```python
from build123d import *

# Parameters (mm, degrees)
F0_W     = 70
F0_H     = 21.5599828357
F0_R     = 2.5
F1_DEPTH = 4
F3_DEPTH = 2
F4_R     = 2


with BuildPart() as f1:
    # F0 (on Top) → F1 (new body)
    with BuildSketch(Plane.XY):
        with Locations((18.8872945234, 0.0549508259)):
            Rectangle(F0_W, F0_H)
        with Locations((-9.1127054766, 0)):
            Circle(F0_R, mode=Mode.SUBTRACT)
    extrude(amount=F1_DEPTH)

    # F2 (on face) → F3 (join)
    with BuildSketch(Plane.XY.offset(4)):
        Polygon((2.2051139605, -3.5713818915), (2.8492078737, -5.2161419195), (3.4717942573, -5.2161419195), (1.4376347458, -0.0226395049), (0.9316418122, -0.0226395049), (-1.1127054766, -5.2161419195), (-0.5037027959, -5.2161419195), (0.1324672907, -3.5713818915), align=None)
        with BuildLine():
            Line((1.4161272162, -1.4274207814), (2.0183380454, -3.0302977254))
            Line((2.0183380454, -3.0302977254), (0.3452786363, -3.0302977254))
            Line((0.3452786363, -3.0302977254), (0.9531493418, -1.4274207814))
            add(Edge.make_bspline(
                [(1.1761484646, -0.6814490963), (1.0980421729, -1.0210416691), (0.9531493418, -1.4274207814)],
                knots=[0, 0, 0, 1, 1, 1], degree=2))
            add(Edge.make_bspline(
                [(1.4161272162, -1.4274207814), (1.2995337661, -1.122919441), (1.1761484646, -0.6814490963)],
                knots=[0, 0, 0, 1, 1, 1], degree=2))
        make_face(mode=Mode.SUBTRACT)
        with BuildLine():
            add(Edge.make_bspline(
                [(7.1009068862, -3.8396600241), (7.1009068862, -4.5222410956), (6.6056677174, -4.9048487277)],
                knots=[0, 0, 0, 1, 1, 1], degree=2))
            add(Edge.make_bspline(
                [(6.7952735706, -2.9770948889), (7.1009068862, -3.3098956104), (7.1009068862, -3.8396600241)],
                knots=[0, 0, 0, 1, 1, 1], degree=2))
            add(Edge.make_bspline(
                [(5.6757500553, -2.3545085053), (6.489640255, -2.6442941675), (6.7952735706, -2.9770948889)],
                knots=[0, 0, 0, 1, 1, 1], degree=2))
            add(Edge.make_bspline(
                [(4.9558138008, -2.0381214249), (5.1912646514, -2.1813162932), (5.6757500553, -2.3545085053)],
                knots=[0, 0, 0, 1, 1, 1], degree=2))
            add(Edge.make_bspline(
                [(4.6213151165, -1.7228663198), (4.7203629503, -1.8949265567), (4.9558138008, -2.0381214249)],
                knots=[0, 0, 0, 1, 1, 1], degree=2))
            add(Edge.make_bspline(
                [(4.5222672828, -1.2825279503), (4.5222672828, -1.5508060828), (4.6213151165, -1.7228663198)],
                knots=[0, 0, 0, 1, 1, 1], degree=2))
            add(Edge.make_bspline(
                [(4.791111403, -0.7131444031), (4.5222672828, -0.918031922), (4.5222672828, -1.2825279503)],
                knots=[0, 0, 0, 1, 1, 1], degree=2))
            add(Edge.make_bspline(
                [(5.5376490757, -0.5082568841), (5.0599555232, -0.5082568841), (4.791111403, -0.7131444031)],
                knots=[0, 0, 0, 1, 1, 1], degree=2))
            add(Edge.make_bspline(
                [(6.7828218429, -0.7765350167), (6.1421238554, -0.5082568841), (5.5376490757, -0.5082568841)],
                knots=[0, 0, 0, 1, 1, 1], degree=2))
            Line((6.7828218429, -0.7765350167), (6.9707297333, -0.2535624544))
            add(Edge.make_bspline(
                [(5.5523647539, 0.0294313563), (6.3232398943, 0.0294313563), (6.9707297333, -0.2535624544)],
                knots=[0, 0, 0, 1, 1, 1], degree=2))
            add(Edge.make_bspline(
                [(4.3632247612, -0.3243109071), (4.812052945, 0.0294313563), (5.5523647539, 0.0294313563)],
                knots=[0, 0, 0, 1, 1, 1], degree=2))
            add(Edge.make_bspline(
                [(3.9143965773, -1.2757360988), (3.9143965773, -0.6780531705), (4.3632247612, -0.3243109071)],
                knots=[0, 0, 0, 1, 1, 1], degree=2))
            add(Edge.make_bspline(
                [(4.2239918063, -2.1988619094), (3.9143965773, -1.845119646), (3.9143965773, -1.2757360988)],
                knots=[0, 0, 0, 1, 1, 1], degree=2))
            add(Edge.make_bspline(
                [(5.254655265, -2.8106945282), (4.5335870352, -2.5526041728), (4.2239918063, -2.1988619094)],
                knots=[0, 0, 0, 1, 1, 1], degree=2))
            add(Edge.make_bspline(
                [(6.0238324426, -3.1395333363), (5.7708359758, -2.9940745176), (5.254655265, -2.8106945282)],
                knots=[0, 0, 0, 1, 1, 1], degree=2))
            add(Edge.make_bspline(
                [(6.3849325451, -3.4564864043), (6.2768289094, -3.284992155), (6.0238324426, -3.1395333363)],
                knots=[0, 0, 0, 1, 1, 1], degree=2))
            add(Edge.make_bspline(
                [(6.4930361808, -3.8962587862), (6.4930361808, -3.6279806536), (6.3849325451, -3.4564864043)],
                knots=[0, 0, 0, 1, 1, 1], degree=2))
            add(Edge.make_bspline(
                [(6.1885348404, -4.5318628851), (6.4930361808, -4.3037698737), (6.4930361808, -3.8962587862)],
                knots=[0, 0, 0, 1, 1, 1], degree=2))
            add(Edge.make_bspline(
                [(5.282954646, -4.7599558966), (5.8840335, -4.7599558966), (6.1885348404, -4.5318628851)],
                knots=[0, 0, 0, 1, 1, 1], degree=2))
            add(Edge.make_bspline(
                [(4.5403788867, -4.6818496048), (4.9150626921, -4.7599558966), (5.282954646, -4.7599558966)],
                knots=[0, 0, 0, 1, 1, 1], degree=2))
            add(Edge.make_bspline(
                [(3.8464780628, -4.4701702344), (4.1656950813, -4.603743313), (4.5403788867, -4.6818496048)],
                knots=[0, 0, 0, 1, 1, 1], degree=2))
            Line((3.8464780628, -4.4701702344), (3.8464780628, -5.0497415588))
            add(Edge.make_bspline(
                [(5.2614471164, -5.2874563598), (4.3422832192, -5.2874563598), (3.8464780628, -5.0497415588)],
                knots=[0, 0, 0, 1, 1, 1], degree=2))
            add(Edge.make_bspline(
                [(6.6056677174, -4.9048487277), (6.1104285486, -5.2874563598), (5.2614471164, -5.2874563598)],
                knots=[0, 0, 0, 1, 1, 1], degree=2))
        make_face()
        with BuildLine():
            add(Edge.make_bspline(
                [(11.0775359147, -3.8396600241), (11.0775359147, -4.5222410956), (10.5822967459, -4.9048487277)],
                knots=[0, 0, 0, 1, 1, 1], degree=2))
            add(Edge.make_bspline(
                [(10.7719025991, -2.9770948889), (11.0775359147, -3.3098956104), (11.0775359147, -3.8396600241)],
                knots=[0, 0, 0, 1, 1, 1], degree=2))
            add(Edge.make_bspline(
                [(9.6523790838, -2.3545085053), (10.4662692835, -2.6442941675), (10.7719025991, -2.9770948889)],
                knots=[0, 0, 0, 1, 1, 1], degree=2))
            add(Edge.make_bspline(
                [(8.9324428293, -2.0381214249), (9.1678936798, -2.1813162932), (9.6523790838, -2.3545085053)],
                knots=[0, 0, 0, 1, 1, 1], degree=2))
            add(Edge.make_bspline(
                [(8.597944145, -1.7228663198), (8.6969919788, -1.8949265567), (8.9324428293, -2.0381214249)],
                knots=[0, 0, 0, 1, 1, 1], degree=2))
            add(Edge.make_bspline(
                [(8.4988963112, -1.2825279503), (8.4988963112, -1.5508060828), (8.597944145, -1.7228663198)],
                knots=[0, 0, 0, 1, 1, 1], degree=2))
            add(Edge.make_bspline(
                [(8.7677404314, -0.7131444031), (8.4988963112, -0.918031922), (8.4988963112, -1.2825279503)],
                knots=[0, 0, 0, 1, 1, 1], degree=2))
            add(Edge.make_bspline(
                [(9.5142781042, -0.5082568841), (9.0365845516, -0.5082568841), (8.7677404314, -0.7131444031)],
                knots=[0, 0, 0, 1, 1, 1], degree=2))
            add(Edge.make_bspline(
                [(10.7594508714, -0.7765350167), (10.1187528839, -0.5082568841), (9.5142781042, -0.5082568841)],
                knots=[0, 0, 0, 1, 1, 1], degree=2))
            Line((10.7594508714, -0.7765350167), (10.9473587617, -0.2535624544))
            add(Edge.make_bspline(
                [(9.5289937823, 0.0294313563), (10.2998689228, 0.0294313563), (10.9473587617, -0.2535624544)],
                knots=[0, 0, 0, 1, 1, 1], degree=2))
            add(Edge.make_bspline(
                [(8.3398537896, -0.3243109071), (8.7886819734, 0.0294313563), (9.5289937823, 0.0294313563)],
                knots=[0, 0, 0, 1, 1, 1], degree=2))
            add(Edge.make_bspline(
                [(7.8910256058, -1.2757360988), (7.8910256058, -0.6780531705), (8.3398537896, -0.3243109071)],
                knots=[0, 0, 0, 1, 1, 1], degree=2))
            add(Edge.make_bspline(
                [(8.2006208347, -2.1988619094), (7.8910256058, -1.845119646), (7.8910256058, -1.2757360988)],
                knots=[0, 0, 0, 1, 1, 1], degree=2))
            add(Edge.make_bspline(
                [(9.2312842934, -2.8106945282), (8.5102160637, -2.5526041728), (8.2006208347, -2.1988619094)],
                knots=[0, 0, 0, 1, 1, 1], degree=2))
            add(Edge.make_bspline(
                [(10.000461471, -3.1395333363), (9.7474650042, -2.9940745176), (9.2312842934, -2.8106945282)],
                knots=[0, 0, 0, 1, 1, 1], degree=2))
            add(Edge.make_bspline(
                [(10.3615615735, -3.4564864043), (10.2534579378, -3.284992155), (10.000461471, -3.1395333363)],
                knots=[0, 0, 0, 1, 1, 1], degree=2))
            add(Edge.make_bspline(
                [(10.4696652092, -3.8962587862), (10.4696652092, -3.6279806536), (10.3615615735, -3.4564864043)],
                knots=[0, 0, 0, 1, 1, 1], degree=2))
            add(Edge.make_bspline(
                [(10.1651638689, -4.5318628851), (10.4696652092, -4.3037698737), (10.4696652092, -3.8962587862)],
                knots=[0, 0, 0, 1, 1, 1], degree=2))
            add(Edge.make_bspline(
                [(9.2595836745, -4.7599558966), (9.8606625285, -4.7599558966), (10.1651638689, -4.5318628851)],
                knots=[0, 0, 0, 1, 1, 1], degree=2))
            add(Edge.make_bspline(
                [(8.5170079151, -4.6818496048), (8.8916917205, -4.7599558966), (9.2595836745, -4.7599558966)],
                knots=[0, 0, 0, 1, 1, 1], degree=2))
            add(Edge.make_bspline(
                [(7.8231070912, -4.4701702344), (8.1423241097, -4.603743313), (8.5170079151, -4.6818496048)],
                knots=[0, 0, 0, 1, 1, 1], degree=2))
            Line((7.8231070912, -4.4701702344), (7.8231070912, -5.0497415588))
            add(Edge.make_bspline(
                [(9.2380761449, -5.2874563598), (8.3189122476, -5.2874563598), (7.8231070912, -5.0497415588)],
                knots=[0, 0, 0, 1, 1, 1], degree=2))
            add(Edge.make_bspline(
                [(10.5822967459, -4.9048487277), (10.0870575771, -5.2874563598), (9.2380761449, -5.2874563598)],
                knots=[0, 0, 0, 1, 1, 1], degree=2))
        make_face()
    extrude(amount=F3_DEPTH)

    # F4
    f4_edges = [f1.edges().sort_by_distance(p)[0] for p in [
        (18.887295, -10.725041, 4),
        (18.887295, 10.834942, 4),
        (53.887295, 0.054951, 4),
    ]]
    fillet(f4_edges, radius=F4_R)


solid = f1.part
```
Input: part model. Units: mm. Frame: model coordinates. A direction names the side the tool comes from. Coordinates: 2 decimals unless noted, no trailing zeros. Order: outer loops, then holes, each group sorted by start corner. A loop starts at its lowest first (then second) coordinate and runs counter-clockwise, first axis right, second up. Notation, with made-up numbers: (67.25, 12.5) - (90.25, 12.5) arc R28 ccw to (90.25, 37.5) - close; hole circle Ø4 at (41.25, 4.5). An arc over 180 degrees is marked (long way). Return JSON: item names as keys, results as strings.
Q1. First-contact query: pin 1 (0.8 mm diameter, centred on x = 1, z = 5, fed in from +Y); pin 2 (8 mm diameter, centred on x = 18.5, y = 0, fed in from +Z); pin 3 (0.5 mm diameter, centred on x = 3, z = 5.5, fed in from -Y); pin 4 (1.8 mm diameter, centred on x = 1, y = -2, fed in from +Z). Flat tips, straight axial feed; report the tip coordinate or a pass-through.
The answers:
{"pin 1": "stops at y = -0.02", "pin 2": "stops at z = 4", "pin 3": "stops at y = -5.22", "pin 4": "stops at z = 6"}
Q2. Cut plane A-A (z = 5). State how many separate pieces and enclosed holes the cut face has, then the cut area to 3 significant figures.
The answers:
{"separate pieces": "3", "enclosed holes": "1", "area": "19.3 mm2"}
Q3. Access query for faces 1 (the flat face through (-0.076, -2.583, 4.986)), 2 (the flat face through (2.52, -4.38, 4.99)), 3 (the flat face through (2.47, -2.66, 4.99)). Directions: +Z, -Z, +X, -X, +Y, -Y. A direction counts if a zero-diameter tool reaches every point of the face in a straight line with its end or side. Return the directions, or none.
The answers:
{"face 1": "+Z, -X, +Y", "face 2": "+Z, -Y", "face 3": "+Z, +Y"}
Q4. Cut plane B-B (y = 1.5). Return loops of the section in (x, z), then the cut area to 3 significant figures.
The answers:
{"outline": "(-16.11, 0) - (-11.11, 0) - (-11.11, 4) - (-16.11, 4) - close; (-7.11, 0) - (53.89, 0) - (53.89, 2) arc R2 ccw to (51.89, 4) - (-7.11, 4) - close", "area": "263 mm2"}
Q5. Draft query along Y for faces 4 (the flat face through (9.5, -2.6, 6)), 5 (the flat face through (1, -3.03, 5)), 6 (the flat face through (-0.19, -4.41, 4.99)). Return one class per face: +Y half, -Y half, draft (parallel to the pull), parting line (faces both ways), or undercut.
The answers:
{"face 4": "draft", "face 5": "undercut", "face 6": "-Y half"}
Q6. Ray query, probe 1 along X at (y, z) = (-1, 5.75); probe 2 along Z at (x, y) = (39.5, -1.75); probe 3 along X at (y, z) = (-4, 4.5). Return the intervals inside material, ascending.
The answers:
{"probe 1": "x = 0.55 to 1.09, 1.27 to 1.82, 3.94 to 4.57, 7.92 to 8.55", "probe 2": "z = 0 to 4", "probe 3": "x = -0.63 to -0.03, 2.37 to 3, 6.49 to 7.09, 10.46 to 11.07"}
Q7. Cut plane C-C (x = 31). Return loops of the section in (y, z).
The answers:
{"outline": "(-10.73, 0) - (10.83, 0) - (10.83, 2) arc R2 ccw to (8.83, 4) - (-8.73, 4) arc R2 ccw to (-10.73, 2) - close"}
